```python
from build123d import *

# Parameters (mm, degrees)
BOSS_EXTRUDE1_DEPTH      = 35
BOSS_EXTRUDE1_DEPTH_BACK = 45
BOSS_EXTRUDE3_DEPTH      = 155
SKETCH5_W                = 5
SKETCH5_H                = 3
BOSS_EXTRUDE5_DEPTH      = 21
CUT_EXTRUDE1_DEPTH       = 10


with BuildPart() as part:
    # Sketch1 → Boss-Extrude1 (new, two sides: drawn at the far end of the back side and taken through both)
    with BuildSketch(Plane.XY.offset(-BOSS_EXTRUDE1_DEPTH_BACK)):
        Polygon((-30, 12), (-30, 10), (-30, -10), (30, -10), (30, 10), (30, 12), (32, 12), (32, -12), (-32, -12), (-32, 12), align=None)
    extrude(amount=BOSS_EXTRUDE1_DEPTH + BOSS_EXTRUDE1_DEPTH_BACK)

    # Sketch3 → Boss-Extrude3 (add)
    with BuildSketch(Plane(origin=(0, 0, -45), x_dir=(-1, 0, 0), z_dir=(0, 0, -1))):
        Polygon((-30, -10), (-30, 12), (-32, 12), (-32, -12), (32, -12), (32, 12), (30, 12), (30, -10), align=None)
    extrude(amount=BOSS_EXTRUDE3_DEPTH)

    # Sketch5 → Boss-Extrude5 (add)
    with BuildSketch(Plane(origin=(0, -10, 0), x_dir=(1, 0, 0), z_dir=(0, 1, 0))):
        with Locations((-27.5, -3.25)):
            Rectangle(SKETCH5_W, SKETCH5_H)
        with Locations((-27.5, 3.25)):
            Rectangle(SKETCH5_W, SKETCH5_H)
        with Locations((27.5, -3.25)):
            Rectangle(SKETCH5_W, SKETCH5_H)
        with Locations((27.5, 3.25)):
            Rectangle(SKETCH5_W, SKETCH5_H)
    extrude(amount=BOSS_EXTRUDE5_DEPTH)

    # Sketch6 → Cut-Extrude1 (cut)
    with BuildSketch(Plane.ZY.offset(32)):
        Polygon((-196.2, 9), (-196.2, -9), (-191.2, -9), (-191.2, 9), (-191.2, 12), (-196.2, 12), align=None)
    extrude(amount=-CUT_EXTRUDE1_DEPTH, mode=Mode.SUBTRACT)


solid = part.part
```
The model under review builds one solid part; all positions refer to its coordinate system, in mm. A direction names the side the tool comes from. Round coordinates to 2 decimals unless told otherwise and drop trailing zeros. Order: outer loops, then holes, each group sorted by start corner. A loop starts at its lowest first (then second) coordinate and runs counter-clockwise, first axis right, second up.
Item 1: Draft analysis for pull direction X (two halves, no side actions). For faces 1 (the flat face through (27, 0, -4.75)), 2 (the flat face through (0, -12, -81)), 3 (the flat face through (-32, 0, -81)), state which applies: released by +X, released by -X, zero draft, split by the parting line, or undercut.
Working result:
face 1: undercut
face 2: zero draft
face 3: released by -X
Item 2: For pin 1 (1.5 mm diameter, centred on x = 28, y = 1.5, fed in from +Z); pin 2 (2.5 mm diameter, centred on x = -27.5, y = -0.5, fed in from -Z); pin 3 (2 mm diameter, centred on x = -31, z = -192.5, fed in from +Y); pin 4 (3 mm diameter, centred on x = 15, y = -7.5, fed in from +Z), all flat-tipped, find the tip position at first contact; note any pin that passes through.
Working result:
pin 1: stops at z = 4.75
pin 2: stops at z = -4.75
pin 3: stops at y = -9
pin 4: passes through
Item 3: Add section D-D, the plane x = -10. State the section outline as (y, z) points.
Working result:
outline: (-12, -200) - (-10, -200) - (-10, 35) - (-12, 35) - close
Item 4: Add section C-C, the plane z = -85. State the section outline as (x, y) points, and give its area (3 significant figures).
Working result:
outline: (-32, -12) - (32, -12) - (32, 12) - (30, 12) - (30, -10) - (-30, -10) - (-30, 12) - (-32, 12) - close
area: 216 mm2
Item 5: Machinability: for faces 4 (the flat face through (-28, 0, 4.75)), 5 (the flat face through (30, 1, -81)), 6 (the flat face through (32, 0, -81)), 7 (the flat face through (-28, 0, -4.75)), which of the approach directions +Z, -Z, +X, -X, +Y, -Y give a long, thin tool a straight path to every point of the face, cutting with its end or side? Answer none if there is none.
Working result:
face 4: +Z, +Y
face 5: +Y
face 6: +Z, -Z, +X, +Y, -Y
face 7: -Z, +Y
Item 6: To check wall thickness, follow probe 1 along X at (y, z) = (9, -72); probe 2 along Y at (x, z) = (3.5, 7). State the ranges of each line that lie inside material, in increasing order.
Working result:
probe 1: x = -32 to -30, 30 to 32
probe 2: y = -12 to -10
Item 7: Add section A-A, the plane y = -0.5. State the section outline as (x, z) points.
Working result:
outline: (-32, -200) - (-30, -200) - (-30, -196.2) - (-32, -196.2) - close; (-32, -191.2) - (-30, -191.2) - (-30, -4.75) - (-25, -4.75) - (-25, -1.75) - (-30, -1.75) - (-30, 1.75) - (-25, 1.75) - (-25, 4.75) - (-30, 4.75) - (-30, 35) - (-32, 35) - close; (25, -4.75) - (30, -4.75) - (30, -200) - (32, -200) - (32, 35) - (30, 35) - (30, 4.75) - (25, 4.75) - (25, 1.75) - (30, 1.75) - (30, -1.75) - (25, -1.75) - close
Item 8: Add section B-B, the plane x = -27. State the section outline as (y, z) points, and give its area (3 significant figures).
Working result:
outline: (-12, -200) - (-10, -200) - (-10, -4.75) - (11, -4.75) - (11, -1.75) - (-10, -1.75) - (-10, 1.75) - (11, 1.75) - (11, 4.75) - (-10, 4.75) - (-10, 35) - (-12, 35) - close
area: 596 mm2
